Verification items for this drawing (mm, ordinates from the low corner). Coordinates: 2 decimals unless noted, no trailing zeros. Order: outer loops, then holes, each group sorted by start corner. A loop starts at its lowest first (then second) coordinate and runs counter-clockwise, first axis right, second up. Notation, with made-up numbers: M 27.5,13 L 43.5,13 A21 ccw 43.5,38 Z; hole C -36,48.25 d8. An arc over 180 degrees is marked long. Return JSON: item names as keys, results as strings. Group by question number.
1. Section check A-A, the plane y = 30. Record the cut outline in (x, z) (3 decimals), plus the area to 3 significant figures.
2. Mould release check, pull along Z, two halves, no side actions. Record for the marked faces 1, 2 and 3: +Z half, -Z half, draft (parallel to the pull), parting line (faces both ways), or undercut.
3. Section check B-B, the plane z = 18.5. Record the cut outline in (x, y).
4. Section check C-C, the plane x = 10. Record the cut outline in (y, z), plus the area to 3 significant figures.
5. Gauge pin test, flat end, axial feed: pin 1 (3.5 mm diameter, centred on x = 70, y = 10, fed in from +Z). Record the tip position at first contact, or that the pin passes through.
6. Section check D-D, the plane z = 4.25. Record the cut outline in (x, y).
7. Material ranges on line 1 along Y through (x, z) = (70, 17.25); line 2 along X through (y, z) = (25.5, 17); line 3 along X through (y, z) = (27.5, 6.75), recorded low to high.
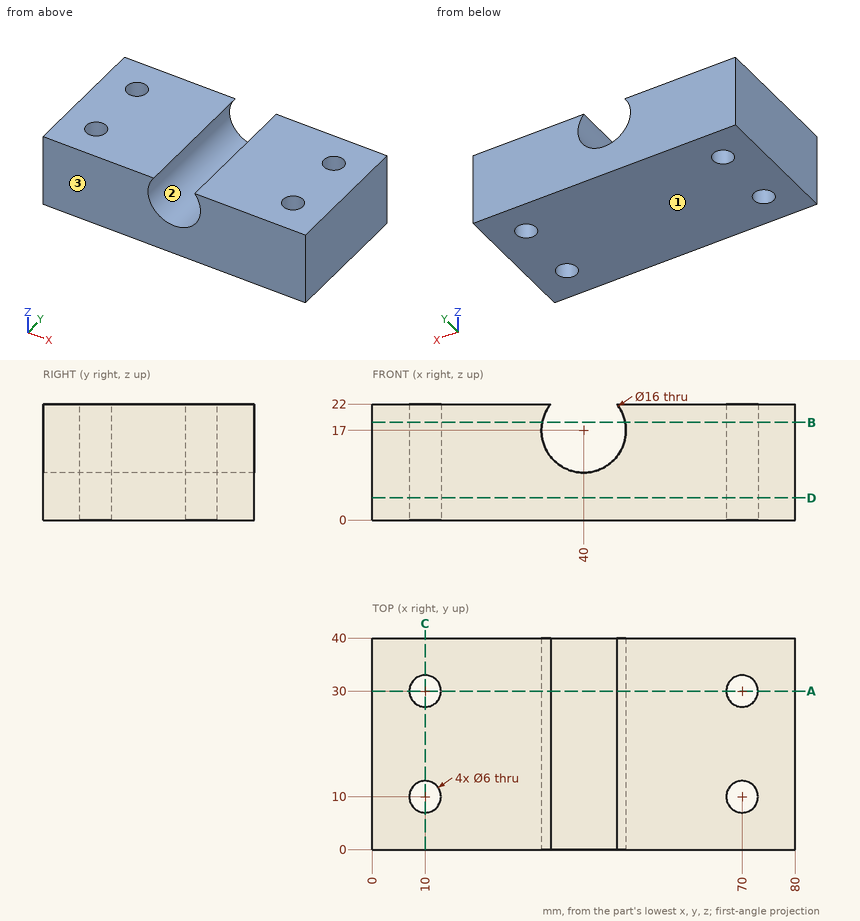
Answers follow:
{
 "1": {"outline": "M 0,0 L 7,0 L 7,22 L 0,22 Z; M 13,0 L 67,0 L 67,22 L 46.245,22 A8 cw long 33.755,22 L 13,22 Z; M 73,0 L 80,0 L 80,22 L 73,22 Z", "area": "1,320 mm^2"},
 "2": {"face 1": "-Z half", "face 2": "undercut", "face 3": "draft"},
 "3": {"outline": "M 0,0 L 32.14,0 L 32.14,40 L 0,40 Z; M 47.86,0 L 80,0 L 80,40 L 47.86,40 Z; hole C 10,10 d6; hole C 10,30 d6; hole C 70,10 d6; hole C 70,30 d6"},
 "4": {"outline": "M 0,0 L 7,0 L 7,22 L 0,22 Z; M 13,0 L 27,0 L 27,22 L 13,22 Z; M 33,0 L 40,0 L 40,22 L 33,22 Z", "area": "616 mm^2"},
 "5": {"pin 1": "through"},
 "6": {"outline": "M 0,0 L 80,0 L 80,40 L 0,40 Z; hole C 10,10 d6; hole C 10,30 d6; hole C 70,10 d6; hole C 70,30 d6"},
 "7": {"line 1": "0 to 7, 13 to 27, 33 to 40", "line 2": "0 to 32, 48 to 80", "line 3": "0 to 8.34, 11.66 to 68.34, 71.66 to 80"}
}
